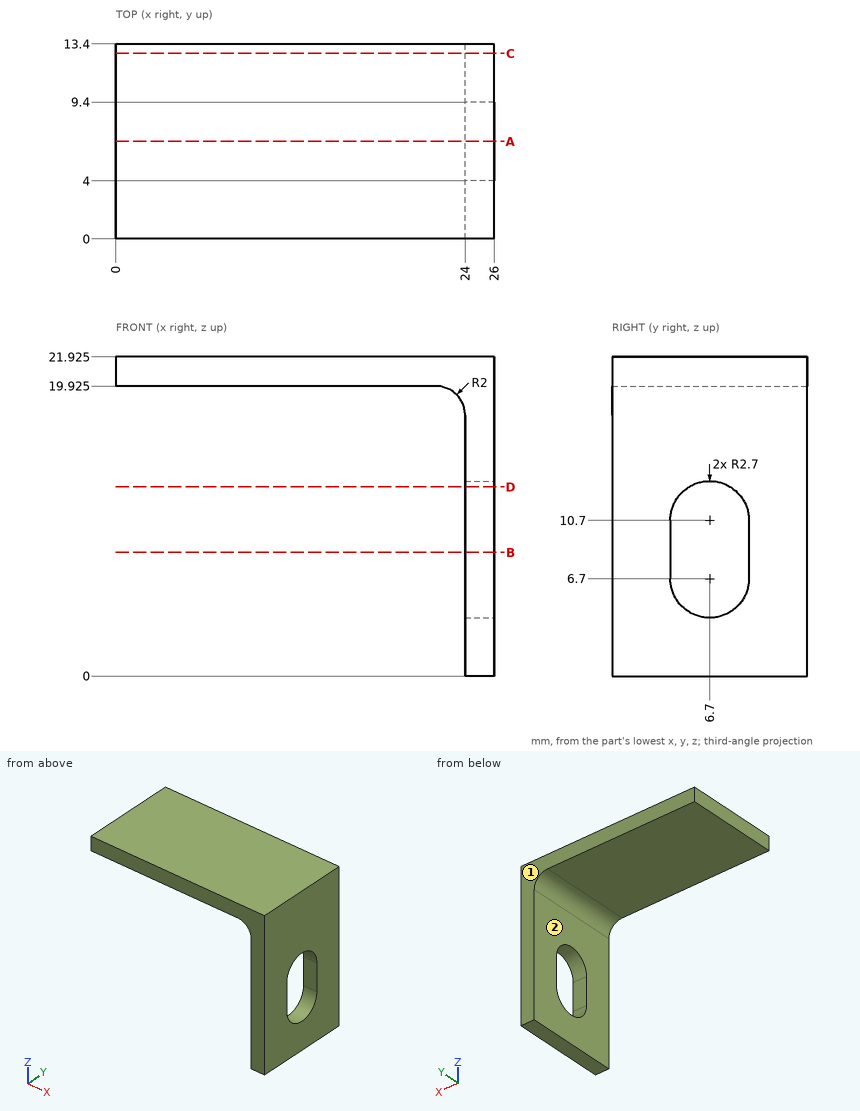
Can you work these out from the drawing? Everything is in mm from the part's minimum corner. A direction names the side the tool comes from. Give positions to 0.01 mm unless a question says otherwise; leave off trailing zeros. Loops run counter-clockwise (first coordinate to the right, second up) from the corner with the lowest first, then second, coordinate; pieces in that order, holes last. Notation, with made-up numbers: (30, 4.25) - (43, 4.25) arc R3 cw to (43, 9.25) - close; hole circle Ø9 at (29.25, 70). An arc over 180 degrees is marked (long way). Answer as a JSON object with one key per item and string values.
Q1. Will these pins go through, and if not, where does the flat tip stop? P1, Ø1, axis at x = 25, z = 8, coming from the -Y side; P2, Ø4, axis at x = 13.5, y = 10, coming from the -Z side (3 decimals).
Geometry says:
{"P1": "y = 0", "P2": "z = 19.925"}
Q2. Imagine slicing it at D-D on z = 13. Write out the boundary of the cut face in (x, y).
Geometry says:
{"outline": "(24, 0) - (26, 0) - (26, 5.29) - (24, 5.29) - close; (24, 8.11) - (26, 8.11) - (26, 13.4) - (24, 13.4) - close"}
Q3. If I drill on L1, parallel to Z at x = 14.5, y = 9.5 (3 decimals); L2, parallel to X at y = 10, z = 3.25; L3, parallel to X at y = 3, z = 18.5, over which ranges is the centre line in solid material (lowest first)?
Geometry says:
{"L1": "19.925 to 21.925", "L2": "24 to 26", "L3": "23.92 to 26"}
Q4. Which directions (+Z, -Z, +X, -X, +Y, -Y) give clear straight access to the entire face, cutting with the end or side of a thin tool? Please do the marked faces 1 and 2.
Geometry says:
{"face 1": "+Z, -Z, +X, -X, +Y", "face 2": "-Z, -X, +Y, -Y"}
Q5. Imagine slicing it at C-C on y = 12.75. Write out the boundary of the cut face in (x, z) (3 decimals).
Geometry says:
{"outline": "(0, 19.925) - (22, 19.925) arc R2 cw to (24, 17.925) - (24, 0) - (26, 0) - (26, 21.925) - (0, 21.925) - close"}
Q6. Imagine slicing it at B-B on z = 8.5. Write out the boundary of the cut face in (x, y).
Geometry says:
{"outline": "(24, 0) - (26, 0) - (26, 4) - (24, 4) - close; (24, 9.4) - (26, 9.4) - (26, 13.4) - (24, 13.4) - close"}
Q7. Imagine slicing it at A-A on y = 6.7. Write out the boundary of the cut face in (x, z) (3 decimals), plus the area to 3 significant figures.
Geometry says:
{"outline": "(0, 19.925) - (22, 19.925) arc R2 cw to (24, 17.925) - (24, 13.4) - (26, 13.4) - (26, 21.925) - (0, 21.925) - close; (24, 0) - (26, 0) - (26, 4) - (24, 4) - close", "area": "73.9 mm²"}
